Work out the finished part from the listing and answer in its coordinate system (mm). A direction names the side the tool comes from. Give positions to 0.01 mm unless a question says otherwise; leave off trailing zeros. Write each loop counter-clockwise with the first axis right and the second up, starting at its lowest first coordinate (ties: lowest second). Pieces come first, ordered by that corner, then holes.
1) Find section A-A (y = 129.5). Determine the outline of the cut face in (x, z) (1 decimal).
2) Find section C-C (z = -36.5). Determine the outline of the cut face in (x, y) (3 decimals), plus the area to 3 significant figures.
3) Find section B-B (x = 31.5). Determine the outline of the cut face in (y, z) (3 decimals).
4) A tool of negligible diameter and unlimited length cuts with its end or side. For faces 1 (the face through (0, 88, -39)), 2 (the face through (55, 90, -3.175)), 3 (the face through (52, 88, 0)), from which of +Z, -Z, +X, -X, +Y, -Y can it reach the whole face along a straight path? Write none if from no direction.
5) Given pin 1 Ø5 at (y, z) = (147.5, -56.5) entering from +X (3 decimals); pin 2 Ø5 at (x, y) = (43, 37.5) entering from -Z (3 decimals); pin 3 Ø1.5 at (y, z) = (141.5, -41) entering from -X; pin 4 Ø1 at (x, y) = (114, 39.5) entering from -Z, each flat-ended and moving along its own axis, determine where each tip first touches the part or whether it passes through.
6) Straight lines are drawn through the part: probe 1 along Z at (x, y) = (47, 39) (3 decimals); probe 2 along X at (y, z) = (71.5, -19.5) (3 decimals); probe 3 along X at (y, z) = (113.5, 8). For each, find the intervals that lie inside material, in ascending order.
Autodesk Inventor part; units mm, degrees
ref_plane "YZ Plane" through (0, 0, 0) normal (1, 0, 0) x (0, 1, 0)
ref_plane "XZ Plane" through (0, 0, 0) normal (0, 1, 0) x (-1, 0, 0)
ref_plane "XY Plane" through (0, 0, 0) normal (0, 0, 1) x (1, 0, 0)
sketch "Sketch1" plane through (0, 0, 0) normal (1, 0, 0) x (0, 1, 0)
  line L0 (0, 0) -> (177.8, 0)
  line L1 (177.8, 0) -> (177.8, -79.375)
  line L2 (177.8, -79.375) -> (0, -79.375)
  line L3 (0, -79.375) -> (0, 0)
  dimension "d0" = 177.8
  dimension "d1" = 79.375
extrude "Extrusion1" add sketch "Sketch1" along normal blind 3.175
sketch "Sketch2" plane through (3.175, 0, 0) normal (1, 0, 0) x (0, 0, -1)
  line L0 (0, 177.8) -> (0, 0)
  line L1 (0, 0) -> (3.175, 0)
  line L2 (3.175, 0) -> (3.175, 177.8)
  line L3 (3.175, 177.8) -> (0, 177.8)
  line L4 (0, 177.8) -> (0, 0)
  dimension "d4" = 3.175
extrude "Extrusion2" add sketch "Sketch2" along normal blind 101.6
sketch "Sketch3" plane through (0, 177.8, 0) normal (0, 1, 0) x (1, 0, 0)
  line L0 (0, 0) -> (104.775, 0)
  line L1 (104.775, 0) -> (126.772, -12.7)
  line L2 (126.772, -12.7) -> (128.3595, -9.9504)
  line L3 (128.3595, -9.9504) -> (105.6257, 3.175)
  line L4 (3.175, 3.175) -> (104.775, 3.175)
  line L5 (105.6257, 3.175) -> (104.775, 3.175)
  line L6 (3.175, 3.175) -> (104.775, 3.175)
  line L7 (104.775, 3.175) -> (104.775, 0)
  line L8 (0, 0) -> (104.775, 0)
  line L9 (104.775, 3.175) -> (104.775, 0)
  dimension "d7" = 3.175
  dimension "d8" = 25.4
  dimension "d9" = 150
extrude "Extrusion3" add sketch "Sketch3" against normal blind 177.8
properties part number "15102898-16-P-0402" material "Aluminum 6061"
Results:
1. outline: (0, -79.4) - (3.2, -79.4) - (3.2, -3.2) - (105.6, -3.2) - (128.4, 10) - (126.8, 12.7) - (104.8, 0) - (0, 0) - close
2. outline: (0, 0) - (3.175, 0) - (3.175, 177.8) - (0, 177.8) - close
2. area: 565 mm2
3. outline: (0, -3.175) - (177.8, -3.175) - (177.8, 0) - (0, 0) - close
4. face 1: +Z, -Z, -X, +Y, -Y
4. face 2: -Z, +X, +Y, -Y
4. face 3: +Z, -X, +Y, -Y
5. pin 1: stops at x = 3.175
5. pin 2: stops at z = -3.175
5. pin 3: stops at x = 0
5. pin 4: stops at z = 1.37
6. probe 1: z = -3.175 to 0
6. probe 2: x = 0 to 3.175
6. probe 3: x = 118.63 to 124.98
